Source: CAD feature listing. Evaluate the final solid. Frame: model axes, mm. A direction names the side the tool comes from. Give positions to 0.01 mm unless a question says otherwise; leave off trailing zeros. Order: outer loops, then holes, each group sorted by start corner. A loop starts at its lowest first (then second) coordinate and runs counter-clockwise, first axis right, second up. Notation, with made-up numbers: (32, 26) -> (46, 26) arc R20 ccw to (46, 49) -> close; hole circle Ø5 at (-1, 59). An arc over 180 degrees is marked (long way). Answer in a Markdown table with one row per item.
Autodesk Inventor part; units mm, degrees
ref_plane "Work Plane1" through (0, 6, 0) normal (0, 1, 0) x (-1, 0, 0)
ref_plane "YZ Plane" through (0, 0, 0) normal (1, 0, 0) x (0, 1, 0)
ref_plane "XY Plane" through (0, 0, 0) normal (0, 0, 1) x (1, 0, 0)
sketch "Sketch1" plane through (0, 0, 0) normal (1, 0, 0) x (0, 1, 0)
  circle A0 centre (0, 0) radius 6
  dimension "d0" = 12
extrude "Extrusion1" add sketch "Sketch1" along normal blind 22.2
ref_plane "Work Plane1" through (0, 6, 0) normal (0, 1, 0) x (-1, 0, 0)
sketch "Sketch2" plane through (0, 6, 0) normal (0, 1, 0) x (-1, 0, 0)
  line L0 (0, 6) -> (0, -6)
  line L1 (-6, 2) -> (-14, 2)
  line L2 (-16, 0) -> (-16, 0)
  line L3 (-14, -2) -> (-6, -2)
  line L4 (-4, 0) -> (-4, 0)
  arc A0 (-4, 0) -> (-6, 2) centre (-6, 0) ccw
  arc A1 (-6, -2) -> (-4, 0) centre (-6, 0) ccw
  arc A2 (-16, 0) -> (-14, -2) centre (-14, 0) ccw
  arc A3 (-14, 2) -> (-16, 0) centre (-14, 0) ccw
  point P0 (0, 0)
  point P1 (-16, -2)
  point P2 (-16, 2)
  point P3 (0, 0)
  point P4 (-16, 0)
  dimension "d3" = 4
  dimension "d4" = 2
  dimension "d5" = 6
  dimension "d6" = 8
extrude "Extrusion2" add sketch "Sketch2" along normal blind 1.6 and the other way blind 1
chamfer "Chamfer1" distance 0.4 angle 45 1 edges at (0, -6, 0)
properties part number "input shaft nmrv-40"
(1) Section query B-B (x = 12). Return the cut outline in (y, z), plus the area to 3 significant figures.
A:
| item | result |
|---|---|
| outline | (5.66, -2) -> (7.6, -2) -> (7.6, 2) -> (5.66, 2) arc R6 ccw (long way) to start |
| area | 120 mm^2 |
(2) Section query C-C (x = 3.25). Return the cut outline in (y, z).
A:
| item | result |
|---|---|
| outline | circle Ø12 at (0, 0) |
(3) First-contact query: pin 1 Ø4 at (x, z) = (8.5, -4.5) entering from -Y; pin 2 Ø4 at (x, y) = (12.5, 2.5) entering from -Z; pin 3 Ø1 at (x, y) = (9.5, 6) entering from -Z. Flat tips, straight axial feed; report the tip coordinate or a pass-through.
A:
| item | result |
|---|---|
| pin 1 | stops at y = -5.45 |
| pin 2 | stops at z = -5.98 |
| pin 3 | stops at z = -2.4 |
(4) Section query A-A (z = 0). Return the cut outline in (x, y), plus the area to 3 significant figures.
A:
| item | result |
|---|---|
| outline | (0, -5.6) -> (0.4, -6) -> (22.2, -6) -> (22.2, 6) -> (16, 6) -> (16, 7.6) -> (4, 7.6) -> (4, 6) -> (0.4, 6) -> (0, 5.6) -> close |
| area | 285 mm^2 |
(5) Ray query, probe 1 along Y at (x, z) = (1.75, 1.5); probe 2 along Y at (x, z) = (5, -3); probe 3 along X at (y, z) = (3.5, 4.5). Return the intervals inside material, ascending.
A:
| item | result |
|---|---|
| probe 1 | y = -5.81 to 5.81 |
| probe 2 | y = -5.2 to 5.2 |
| probe 3 | x = 0.1 to 22.2 |
(6) Access query for faces 1 (the cylindrical face through (4, 7, 0)), 2 (the cylindrical face through (16, 7, 0)), 3 (the flat face through (10, 7, 2)), 4 (the flat face through (10, 7, -2)). Directions: +Z, -Z, +X, -X, +Y, -Y. A direction counts if a zero-diameter tool reaches every point of the face in a straight line with its end or side. Return the directions, or none.
A:
| item | result |
|---|---|
| face 1 | -X, +Y |
| face 2 | +X, +Y |
| face 3 | +Z, +X, -X, +Y |
| face 4 | -Z, +X, -X, +Y |
